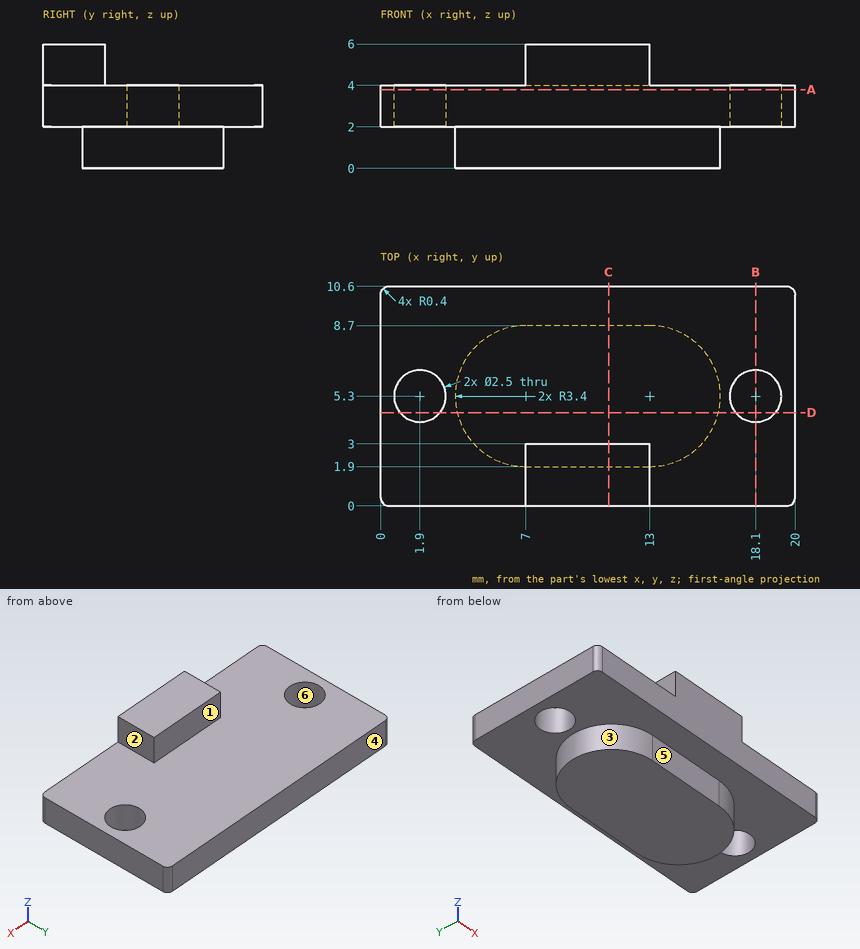
Study the drawing (mm; zero at the part's minimum x, y, z) and answer. A direction names the side the tool comes from. Give positions to 0.01 mm unless a question says otherwise; leave off trailing zeros. Write each loop counter-clockwise with the first axis right and the second up, starting at its lowest first coordinate (ties: lowest second). Pieces come first, ordered by that corner, then holes. Notation, with made-up numbers: (53.5, 8.25) -> (103.5, 8.25) arc R12 cw to (103.5, 16.25) -> close; hole circle Ø4 at (0, -2.75). An arc over 180 degrees is marked (long way). Write item = value, one per line. Start each with the question number.
1) Each of these flat-tipped pins is pushed along its axis until it touches: pin 1 (2 mm diameter, centred on x = 1.9, y = 5.3, fed in from -Z); pin 2 (3 mm diameter, centred on x = 9, y = 3.5, fed in from +Z); pin 3 (3 mm diameter, centred on x = 18.1, y = 5.3, fed in from -Z); pin 4 (0.6 mm diameter, centred on x = 11.5, z = 0.5, fed in from +Y). Where does it stop, or does it pass through?
2) The part is cut by section B-B, the plane x = 18.1. Determine the outline of the cut face in (y, z), and give its area (3 significant figures).
3) The part is cut by section A-A, the plane z = 3.8. Determine the outline of the cut face in (x, y).
4) Which of the six approach directions +Z, -Z, +X, -X, +Y, -Y give full straight-line access (tool end or side, diameter ignored) to the marked faces 1, 2 and 3?
5) Determine the mould class of the marked faces 4, 5 and 6 for opening direction Y: +Y half, -Y half, draft (parallel to the pull), parting line (faces both ways), or undercut.
6) Straight lines are drawn through the part: line 1 along Y through (x, z) = (1.9, 3.15); line 2 along X through (y, z) = (6, 2.55); line 3 along Z through (x, y) = (8, 8.75). For each, find the intervals that lie inside material, in ascending order.
7) The part is cut by section D-D, the plane y = 4.5. Determine the outline of the cut face in (x, z), and give its area (3 significant figures).
8) The part is cut by section C-C, the plane x = 11. Determine the outline of the cut face in (y, z), and give its area (3 significant figures).
Solutions:
q1.pin_1 = through
q1.pin_2 = 6
q1.pin_3 = 2
q1.pin_4 = 8.7
q2.outline = (0, 2) -> (4.05, 2) -> (4.05, 4) -> (0, 4) -> close; (6.55, 2) -> (10.6, 2) -> (10.6, 4) -> (6.55, 4) -> close
q2.area = 16.2 mm²
q3.outline = (0, 0.4) arc R0.4 ccw to (0.4, 0) -> (19.6, 0) arc R0.4 ccw to (20, 0.4) -> (20, 10.2) arc R0.4 ccw to (19.6, 10.6) -> (0.4, 10.6) arc R0.4 ccw to (0, 10.2) -> close; hole circle Ø2.5 at (1.9, 5.3); hole circle Ø2.5 at (18.1, 5.3)
q4.face_1 = +Z, +X, -X, +Y
q4.face_2 = +Z, +X, +Y, -Y
q4.face_3 = -Z, -X
q5.face_4 = +Y half
q5.face_5 = -Y half
q5.face_6 = undercut
q6.line_1 = 0 to 4.05, 6.55 to 10.6
q6.line_2 = 0 to 0.86, 2.94 to 17.06, 19.14 to 20
q6.line_3 = 2 to 4
q7.outline = (0, 2) -> (0.94, 2) -> (0.94, 4) -> (0, 4) -> close; (2.86, 2) -> (3.7, 2) -> (3.7, 0) -> (16.3, 0) -> (16.3, 2) -> (17.14, 2) -> (17.14, 4) -> (2.86, 4) -> close; (19.06, 2) -> (20, 2) -> (20, 4) -> (19.06, 4) -> close
q7.area = 57.5 mm²
q8.outline = (0, 2) -> (1.9, 2) -> (1.9, 0) -> (8.7, 0) -> (8.7, 2) -> (10.6, 2) -> (10.6, 4) -> (3, 4) -> (3, 6) -> (0, 6) -> close
q8.area = 40.8 mm²
